```python
from build123d import *

# Parameters (mm, degrees)
F0_R            = 2.5000000706
F0_R_2          = 2.5000000298
F0_W            = 4.9999998882
F0_H            = 5.2
F1_DEPTH        = 100
F3_DEPTH        = 35
F6_D            = 4.4
F6_DEPTH        = 40
F6_TIP          = 1.3218933619
F5_W            = 10
F5_H            = 6
F7_DEPTH        = 10
F9_D            = 5.5
F9_DEPTH        = 40
F9_TIP          = 1.6523667023
F11_D           = 3.3
F11_DEPTH       = 20
F11_START       = 1.4999997
F11_CBORE_D     = 6.5
F11_CBORE_DEPTH = 3
F11_TIP         = 0.9914200214
F12_DEPTH       = 4


# Not quite as in the source:
# - after a boolean that leaves OpenCascade's solid faulty, fix() repairs it
# - ends of sketch curves that miss each other by under 0.0002 mm in the source are joined
# - a feature names something its author has since deleted; it is built from what else it names


with BuildPart() as f1:
    # F0 (on Front) → F1 (new body)
    with BuildSketch(Plane.XZ):
        Polygon((-38.4980148883, 4.2457092745), (-38.4980148883, -5.7542903855), (-8.4980155588, -5.7542903855), (-8.4980155588, 4.2457092745), (-15.6109269008, 4.2457092745), (-20.5109269008, 4.2457092745), (-25.510926789, 4.2457092745), (-30.410926789, 4.2457092745), align=None)
        with Locations((-30.9980151824, -0.7542907016)):
            Circle(F0_R, mode=Mode.SUBTRACT)
        with Locations((-15.9980151584, -0.7062930843)):
            Circle(F0_R_2, mode=Mode.SUBTRACT)
        with Locations((-23.0109268449, 6.8457092745)):
            Rectangle(F0_W, F0_H)
        with Locations((-30.9980151824, -0.7542907016)):
            Circle(F0_R)
        with Locations((-15.9980151584, -0.7062930843)):
            Circle(F0_R_2)
        Polygon((-30.410926789, 12.2457092745), (-30.410926789, 9.4457092745), (-25.510926789, 9.4457092745), (-20.5109269008, 9.4457092745), (-15.6109269008, 9.4457092745), (-15.6109269008, 12.2457092745), align=None)
    extrude(amount=F1_DEPTH)

    # F2 (on face) → F3 (join)
    with BuildSketch(Plane(origin=(0, 0, 0), x_dir=(-1, 0, 0), z_dir=(0, 1, 0))):
        Polygon((8.4980155588, 10.7457096145), (8.4980155588, 4.2457092745), (20.5109269008, 4.2457092745), (20.5109269008, 9.4457092745), (15.6109269008, 9.4457092745), (15.6109269008, 10.7457096145), align=None)
        Polygon((25.510926789, 4.2457092745), (38.4980148883, 4.2457092745), (38.4980155588, 10.7457096145), (30.410926789, 10.7457096145), (30.410926789, 9.4457092745), (25.510926789, 9.4457092745), align=None)
        Polygon((8.4980155588, 4.2457092745), (8.4980155588, -5.7542903855), (38.4980155588, -5.7542903855), (38.4980155588, 4.2457092745), (25.510926789, 4.2457092745), (25.510926789, 9.4457092745), (30.410926789, 9.4457092745), (30.410926789, 10.7457096145), (15.6109269008, 10.7457096145), (15.6109269008, 9.4457092745), (20.5109269008, 9.4457092745), (20.5109269008, 4.2457092745), align=None)
    extrude(amount=F3_DEPTH)

    # F4: union 

    # F6
    with Locations(Plane(origin=(0, 0, -5.7542903855), x_dir=(1, 0, 0), z_dir=(0, 0, -1))):
        with Locations((-15.4980155588, -20), (-31.4980148883, -20)):
            Hole(F6_D / 2, depth=F6_DEPTH)
            with Locations((0, 0, -(F6_DEPTH + F6_TIP / 2))):  # 118° drill point
                Cone(0, F6_D / 2, F6_TIP, mode=Mode.SUBTRACT)

    # F5 (on face) → F7 (cut)
    with BuildSketch(Plane(origin=(0, 0, -5.7542903855), x_dir=(1, 0, 0), z_dir=(0, 0, -1))):
        with Locations((-15.9980155588, 88)):
            Rectangle(F5_W, F5_H)
        with Locations((-30.9980148883, 88)):
            Rectangle(F5_W, F5_H)
    extrude(amount=-F7_DEPTH, mode=Mode.SUBTRACT)

    add(f1.part.fix(), mode=Mode.REPLACE)

    # F9
    with Locations(Plane.XZ.offset(100)):
        with Locations((-30.9980151824, -0.7542907016), (-15.9980151584, -0.7062930843)):
            Hole(F9_D / 2, depth=F9_DEPTH)
            with Locations((0, 0, -(F9_DEPTH + F9_TIP / 2))):  # 118° drill point
                Cone(0, F9_D / 2, F9_TIP, mode=Mode.SUBTRACT)

    # F11
    # its depths count from where the whole tool has entered the part; down to there all is cleared
    with Locations(Plane.XY.offset(12.2457092745)):
        with Locations((-23.0109268449, 0, -F11_START), (-23.0109268449, -70, 0)):
            CounterBoreHole(F11_D / 2, F11_CBORE_D / 2, F11_CBORE_DEPTH, depth=F11_DEPTH)
            with Locations((0, 0, -(F11_DEPTH + F11_TIP / 2))):  # 118° drill point
                Cone(0, F11_D / 2, F11_TIP, mode=Mode.SUBTRACT)

    # F5 (on face) → F12 (cut)
    with BuildSketch(Plane(origin=(0, 0, -5.7542903855), x_dir=(1, 0, 0), z_dir=(0, 0, -1))):
        Polygon((-18.9980155588, -17.9792740578), (-18.9980155588, -22.0207259422), (-15.4980155588, -24.0414518843), (-11.9980155588, -22.0207259422), (-11.9980155588, -17.9792740578), (-15.4980155588, -15.9585481157), align=None)
        Polygon((-31.4247349717, -24.0407874712), (-27.9619503287, -21.9569314662), (-28.0352302453, -17.9161439951), (-31.5712948049, -15.9592125288), (-35.0340794479, -18.0430685338), (-34.9607995313, -22.0838560049), align=None)
    extrude(amount=-F12_DEPTH, mode=Mode.SUBTRACT)


solid = f1.part
```
Verification items for the finished model (mm, model axes). A direction names the side the tool comes from. Give positions to 0.01 mm unless a question says otherwise; leave off trailing zeros. Write each loop counter-clockwise with the first axis right and the second up, starting at its lowest first coordinate (ties: lowest second). Pieces come first, ordered by that corner, then holes. Notation, with made-up numbers: M 48.5,83 L 61.5,83 A30 cw 61.5,117 Z; hole C 9,36.25 d10. An arc over 180 degrees is marked long. One line per question, with ' | ' between items.
1) Section check B-B on y = -55.5. Enter the section's corners in (x, z), plus the area to 3 significant figures.
Result:
outline: M -38.5,-5.75 L -8.5,-5.75 L -8.5,4.25 L -20.51,4.25 L -20.51,9.45 L -15.61,9.45 L -15.61,12.25 L -30.41,12.25 L -30.41,9.45 L -25.51,9.45 L -25.51,4.25 L -38.5,4.25 Z | area: 367 mm2
2) Section check C-C on y = -70. Enter the section's corners in (x, z).
Result:
outline: M -38.5,-5.75 L -24.66,-5.75 L -24.66,9.25 L -25.51,9.25 L -25.51,4.25 L -38.5,4.25 Z; M -30.41,9.45 L -26.26,9.45 L -26.26,12.25 L -30.41,12.25 Z; M -21.36,-5.75 L -8.5,-5.75 L -8.5,4.25 L -20.51,4.25 L -20.51,9.25 L -21.36,9.25 Z; M -19.76,9.45 L -15.61,9.45 L -15.61,12.25 L -19.76,12.25 Z; hole C -31,-0.75 d5.5; hole C -16,-0.71 d5.5
3) Gauge pin test, flat ends, axial feed: pin 1 Ø2 at (y, z) = (-28.5, 10.5) entering from -X; pin 2 Ø5.5 at (x, y) = (-31.5, 20) entering from +Z; pin 3 Ø3.5 at (x, z) = (-31, -0.75) entering from -Y; pin 4 Ø4 at (x, y) = (-15.5, 20) entering from -Z. Record the tip position at first contact, or that the pin passes through.
Result:
pin 1: stops at x = -30.41 | pin 2: stops at z = 10.75 | pin 3: stops at y = -59.4 | pin 4: passes through
4) Mould release check, pull along X, two halves, no side actions. Record for faces 1 (the flat face through (-18, -49, 9.446)), 2 (the flat face through (-29.718, 23.013, -3.782)), 3 (the flat face through (-25.511, -49, 7)): released by +X, released by -X, zero draft, split by the parting line, or undercut.
Result:
face 1: zero draft | face 2: undercut | face 3: released by -X
5) Thickness scan on line 1 along X through (y, z) = (20, 7.75); line 2 along Y through (x, z) = (-16.5, 2.5); line 3 along Y through (x, z) = (-32.25, 10.25). Record the ranges inside material, lowest first. Write a range as [from, to].
Result:
line 1: x = [-38.5, -33.7], [-29.3, -17.7], [-13.3, -8.5] | line 2: y = [-100, -91], [-85, 18.04], [21.96, 35] | line 3: y = [0, 17.93], [22.07, 35]
6) Section check A-A on y = -88.5. Enter the section's corners in (x, z).
Result:
outline: M -38.5,-5.75 L -36,-5.75 L -36,4.25 L -38.5,4.25 Z; M -30.41,9.45 L -25.51,9.45 L -25.51,4.25 L -26,4.25 L -26,-5.75 L -21,-5.75 L -21,4.25 L -20.51,4.25 L -20.51,9.45 L -15.61,9.45 L -15.61,12.25 L -30.41,12.25 Z; M -11,-5.75 L -8.5,-5.75 L -8.5,4.25 L -11,4.25 Z
7) Section check D-D on y = 20. Enter the section's corners in (x, z), plus the area to 3 significant figures.
Result:
outline: M -38.5,-5.75 L -35,-5.75 L -35,-1.75 L -33.7,-1.75 L -33.7,10.75 L -38.5,10.75 L -38.5,4.25 Z; M -29.3,-1.75 L -28,-1.75 L -28,-5.75 L -19,-5.75 L -19,-1.75 L -17.7,-1.75 L -17.7,10.75 L -29.3,10.75 Z; M -13.3,-1.75 L -12,-1.75 L -12,-5.75 L -8.5,-5.75 L -8.5,10.75 L -13.3,10.75 Z | area: 329 mm2
8) Set-up check for faces 4 (the flat face through (-10.998, -88, -1)), 5 (the flat face through (-28, -49, 9.446)), 6 (the flat face through (-25.998, -88, -1)), 7 (the cylindrical face through (-33.62, -95.44, 0.07)): record each of +Z, -Z, +X, -X, +Y, -Y from which the full face is reachable in a straight line by a thin tool's end or side.
Result:
face 4: +Z, -Z | face 5: -X, -Y | face 6: -Z | face 7: -Y
